Autodesk Inventor part; units mm, degrees
ref_plane "YZ Plane" through (0, 0, 0) normal (1, 0, 0) x (0, 1, 0)
ref_plane "XZ Plane" through (0, 0, 0) normal (0, 1, 0) x (-1, 0, 0)
ref_plane "XY Plane" through (0, 0, 0) normal (0, 0, 1) x (1, 0, 0)
sketch "Sketch2" plane through (0, 0, 0) normal (0, 0, 1) x (1, 0, 0)
  line L0 (2.4, 4.4) -> (2.4, 0)
  line L1 (2.4, 0) -> (2.8, 0)
  line L2 (2.8, 0) -> (2.8, 1.2)
  line L3 (2.8, 1.2) -> (3.2, 1.2)
  line L4 (3.2, 1.2) -> (3.2, 4.4)
  arc A0 (3.2, 4.4) -> (0, 7.6) centre (0, 4.4) ccw
  line L5 (0, 7.6) -> (0, -3.6)
  line L6 (0, -3.6) -> (1.6, -3.6)
  line L7 (1.6, -3.6) -> (1.6, 6.1889)
  arc A1 (2.4, 4.4) -> (1.6, 6.1889) centre (0, 4.4) ccw
  point P0 (0, 0)
  dimension "d0" = 3.6
  dimension "d1" = 6.4
  dimension "d2" = 5.6
  dimension "d3" = 1.2
  dimension "d4" = 3.2
  dimension "d5" = 6.4
  dimension "d6" = 4.8
revolve "Revolution1" add sketch "Sketch2" angle 360 about axis through (0, 7.6, 0) along (0, -1, 0)
equation "\"d4\" = rd"
properties part number "58176-TransRed" material "ABS Plastic"
Design review of the part built by this model. Coordinates are the model's own, in mm. A direction names the side the tool comes from. Coordinates: 2 decimals unless noted, no trailing zeros. Order: outer loops, then holes, each group sorted by start corner. A loop starts at its lowest first (then second) coordinate and runs counter-clockwise, first axis right, second up.
Item 1: For pin 1 Ø1 at (y, z) = (5, -0.5) entering from -X; pin 2 Ø3 at (x, y) = (1, -2.5) entering from +Z; pin 3 Ø1.5 at (y, z) = (5.5, 1) entering from -X, all flat-tipped, find the tip position at first contact; note any pin that passes through.
Item 2: Take a section at B-B, the plane y = -0.75. Write out the cut boundary in (x, z), then the cut area to 3 significant figures.
Item 3: The part is to be moulded in two halves that separate along Z. For faces 1 (the cylindrical face through (-1.27, 1.36, 0.97)), 2 (the flat face through (0, 1.2, -3)), 3 (the cylindrical face through (-2.539, 2.822, 1.947)), say which applies: pulls with the +Z half, pulls with the -Z half, needs draft (parallel to the pull), parting line crosses it, or undercut.
Item 4: For line 1 (Z direction, x = 0, y = 2.1); line 2 (Z direction, x = 0, y = 0.25); line 3 (X direction, y = 2.5, z = 0.5), list the stretches that pass through material, from the lowest coordinate up.
Item 5: Take a section at C-C, the plane x = 3. Write out the cut boundary in (y, z), then the cut area to 3 significant figures.
Item 6: For faces 4 (the cylindrical face through (1.29, 2.169, 2.024)), 5 (the flat face through (0, -3.6, 0)), list the 3-axis set-ups (+Z, -Z, +X, -X, +Y, -Y) from which the entire face can be reached by the end or side of a thin tool; tool diameter is ignored.
Item 7: Take a section at A-A, the plane y = 3.5. Write out the cut boundary in (x, z), then the cut area to 3 significant figures.
The answers:
1. pin 1: stops at x = -3.19
1. pin 2: stops at z = 1.6
1. pin 3: stops at x = -3.11
2. outline: circle Ø3.2 at (0, 0)
2. area: 8.04 mm2
3. face 1: undercut
3. face 2: needs draft
3. face 3: parting line crosses it
4. line 1: z = -3.2 to -2.4, -1.6 to 1.6, 2.4 to 3.2
4. line 2: z = -2.8 to -2.4, -1.6 to 1.6, 2.4 to 2.8
4. line 3: x = -3.16 to -2.35, -1.52 to 1.52, 2.35 to 3.16
5. outline: (1.2, -1.11) - (4.4, -1.11) arc R1.11 ccw to (4.4, 1.11) - (1.2, 1.11) - close
5. area: 9.07 mm2
6. face 4: -Y
6. face 5: +Z, -Z, +X, -X, -Y
7. outline: circle Ø6.4 at (0, 0); circle Ø3.2 at (0, 0); hole circle Ø4.8 at (0, 0)
7. area: 22.1 mm2
